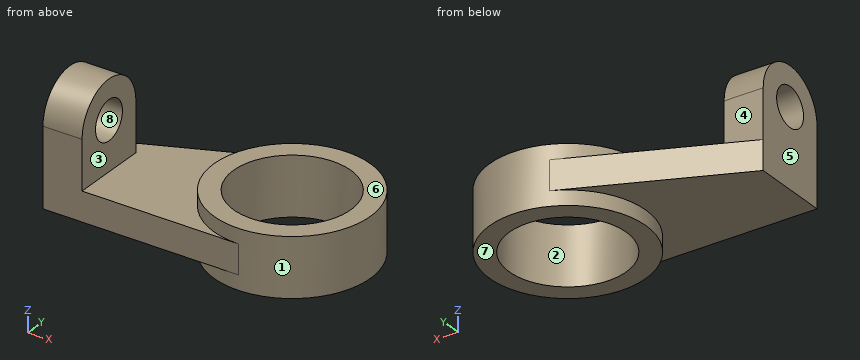
from build123d import *

# Parameters (mm, degrees)
SKETCH1_R           = 50.8
SKETCH1_R_2         = 38.1
BOSS_EXTRUDE1_DEPTH = 19.05
BOSS_EXTRUDE2_DEPTH = 9.525
SKETCH3_W           = 25.4
SKETCH3_H           = 50.8
BOSS_EXTRUDE3_DEPTH = 31.75
SKETCH4_R           = 25.4
SKETCH4_R_2         = 12.7
BOSS_EXTRUDE5_DEPTH = 25.4
SKETCH5_R           = 12.7
CUT_EXTRUDE1_DEPTH  = 197.56814499


with BuildPart() as part:
    # Sketch1 → Boss-Extrude1 (new, symmetric)
    with BuildSketch(Plane.XY):
        with Locations(Location((0, 0, 0), (0, 0, 180))):
            Circle(SKETCH1_R)
        with Locations(Location((0, 0, 0), (0, 0, 180))):
            Circle(SKETCH1_R_2, mode=Mode.SUBTRACT)
    extrude(amount=BOSS_EXTRUDE1_DEPTH, both=True)

    # Sketch2 → Boss-Extrude2 (add, symmetric)
    with BuildSketch(Plane.XY):
        with BuildLine():
            Line((0, -50.8), (-127, -50.8))
            Line((-127, -50.8), (-127, 0))
            Line((-127, 0), (-20.32, 46.558969061))
            ThreePointArc((-20.32, 46.558969061), (-49.728440697, -10.378929899), (0, -50.8))
        make_face()
    extrude(amount=BOSS_EXTRUDE2_DEPTH, both=True)

    # Sketch3 → Boss-Extrude3 (add)
    with BuildSketch(Plane.XY.offset(9.525)):
        with Locations((-114.3, -25.4)):
            Rectangle(SKETCH3_W, SKETCH3_H)
    extrude(amount=BOSS_EXTRUDE3_DEPTH)

    # Sketch4 → Boss-Extrude5 (add)
    with BuildSketch(Plane.ZY.offset(127)):
        with Locations((41.275, -25.4)):
            Circle(SKETCH4_R)
        with Locations((41.275, -25.4)):
            Circle(SKETCH4_R_2, mode=Mode.SUBTRACT)
    extrude(amount=-BOSS_EXTRUDE5_DEPTH)

    # Sketch5 → Cut-Extrude1 (cut, through all)
    with BuildSketch(Plane.ZY.offset(127)):
        with Locations((41.275, -25.4)):
            Circle(SKETCH5_R)
    extrude(amount=-CUT_EXTRUDE1_DEPTH, mode=Mode.SUBTRACT)


solid = part.part
Verification items for the finished model (mm, model axes). Face numbers are marked on the shaded views. A direction names the side the tool comes from. Round coordinates to 2 decimals unless told otherwise and drop trailing zeros. Loops run counter-clockwise (first coordinate to the right, second up) from the corner with the lowest first, then second, coordinate; pieces in that order, holes last. Notation, with made-up numbers: (-24, -37.75) - (11, -37.75) arc R15 ccw to (11, -12.75) - close; hole circle Ø10 at (19.25, 74). An arc over 180 degrees is marked (long way). Answer in a Markdown table with one row per item. Add a question column.
Q1. Section check C-C on y = -32. Enter the section's corners in (x, z) (3 decimals).
Q2. Tool access check on the marked faces 1, 2, 3 and 4. Record the directions out of +Z, -Z, +X, -X, +Y, -Y that give a thin tool (end or side, any length) a straight path to the whole face; none if there is none.
Q3. Gauge pin test, flat ends, axial feed: pin 1 (2 mm diameter, centred on x = -58, y = -1, fed in from +Z) (3 decimals); pin 2 (20.5 mm diameter, centred on x = -120.5, z = 22, fed in from +Y); pin 3 (2 mm diameter, centred on x = -63.5, y = 12.5, fed in from -Z) (3 decimals). Record the tip position at first contact, or that the pin passes through.
Q4. Section check D-D on y = 11.5. Enter the section's corners in (x, z) (3 decimals).
Q5. Section check A-A on x = -34.5. Enter the section's corners in (y, z) (3 decimals), plus the area to 3 significant figures.
Q6. Section check B-B on z = 6. Enter the section's corners in (x, y).
Q7. Release check for a two-part mould opening along Z. For the marked faces 5, 6, 7 and 8 record: pulls with the +Z half, pulls with the -Z half, needs draft (parallel to the pull), parting line crosses it, or undercut.
Q8. Material ranges on line 1 (Z direction, x = -109, y = -25.4) (3 decimals); line 2 (Z direction, x = -100.5, y = -21.5) (3 decimals); line 3 (Z direction, x = 6, y = 40), recorded low to high.
Found:
| question | item | result |
|---|---|---|
| 1 | outline | (-127, -9.525) - (-39.454, -9.525) - (-39.454, -19.05) - (-20.679, -19.05) - (-20.679, 19.05) - (-39.454, 19.05) - (-39.454, 9.525) - (-101.6, 9.525) - (-101.6, 30.425) - (-127, 30.425) - close; (-127, 52.125) - (-101.6, 52.125) - (-101.6, 65.803) - (-127, 65.803) - close; (20.679, -19.05) - (39.454, -19.05) - (39.454, 19.05) - (20.679, 19.05) - close |
| 2 | face 1 | none |
| 2 | face 2 | +Z, -Z |
| 2 | face 3 | +Z, +Y, -Y |
| 2 | face 4 | +Z, -X, +Y |
| 3 | pin 1 | stops at z = 9.525 |
| 3 | pin 2 | stops at y = 0 |
| 3 | pin 3 | stops at z = -9.525 |
| 4 | outline | (-100.65, -9.525) - (-49.481, -9.525) - (-49.481, -19.05) - (-36.323, -19.05) - (-36.323, 19.05) - (-49.481, 19.05) - (-49.481, 9.525) - (-100.65, 9.525) - close; (36.323, -19.05) - (49.481, -19.05) - (49.481, 19.05) - (36.323, 19.05) - close |
| 5 | outline | (-50.8, -9.525) - (-37.288, -9.525) - (-37.288, -19.05) - (-16.167, -19.05) - (-16.167, 19.05) - (-37.288, 19.05) - (-37.288, 9.525) - (-50.8, 9.525) - close; (16.167, -19.05) - (37.288, -19.05) - (37.288, -9.525) - (40.37, -9.525) - (40.37, 9.525) - (37.288, 9.525) - (37.288, 19.05) - (16.167, 19.05) - close |
| 5 | area | 1,930 mm² |
| 6 | outline | (-127, -50.8) - (0, -50.8) arc R50.8 ccw (long way) to (-20.32, 46.56) - (-127, 0) - close; hole circle Ø76.2 at (0, 0) |
| 7 | face 5 | needs draft |
| 7 | face 6 | pulls with the +Z half |
| 7 | face 7 | pulls with the -Z half |
| 7 | face 8 | undercut |
| 8 | line 1 | z = -9.525 to 28.575, 53.975 to 66.675 |
| 8 | line 2 | z = -9.525 to 9.525 |
| 8 | line 3 | z = -19.05 to 19.05 |
